The model under review builds one solid part; all positions refer to its coordinate system, in mm. Coordinates: 2 decimals unless noted, no trailing zeros. Loops run counter-clockwise (first coordinate to the right, second up) from the corner with the lowest first, then second, coordinate; pieces in that order, holes last. Notation, with made-up numbers: (50, 80) - (98, 80) arc R19 cw to (98, 88) - close; hole circle Ø1 at (32, 56). An arc over 180 degrees is marked (long way). One line per item, written item: value. Start each with the question number.
1. We need section A-A, the plane z = 111. Give the boundary of the cut face in (x, y).
2. We need section C-C, the plane y = -13.5. Give the boundary of the cut face in (x, z), then the cut area to 3 significant figures.
3. We need section B-B, the plane x = -7.25. Give the boundary of the cut face in (y, z), then the cut area to 3 significant figures.
4. Insertion check: P1, Ø4, axis at y = -15.5, z = 39, coming from the -X side. The pin has a flat end and moves straight along its axis. Give the tip position at first contact, or say it passes through.
5. To check wall thickness, follow line 1 (Y direction, x = 6.5, z = 116); line 2 (X direction, y = -5, z = 13.5); line 3 (X direction, y = -9, z = 130.5). State the ranges of each line that lie inside material, in increasing order.
Autodesk Inventor part; units mm, degrees
ref_plane "YZ Plane" through (0, 0, 0) normal (1, 0, 0) x (0, 1, 0)
ref_plane "XZ Plane" through (0, 0, 0) normal (0, 1, 0) x (-1, 0, 0)
ref_plane "XY Plane" through (0, 0, 0) normal (0, 0, 1) x (1, 0, 0)
sketch "Sketch1" plane through (0, 0, 0) normal (0, 0, 1) x (1, 0, 0)
  line L0 (-4.3602, -2.3462) -> (5.1648, -2.3462)
  line L1 (5.1648, -2.3462) -> (9.9273, -10.5951)
  line L2 (9.9273, -10.5951) -> (5.1648, -18.844)
  line L3 (5.1648, -18.844) -> (-4.3602, -18.844)
  line L4 (-4.3602, -18.844) -> (-9.1227, -10.5951)
  line L5 (-9.1227, -10.5951) -> (-4.3602, -2.3462)
  point P0 (0, 0)
  dimension "d0" = 9.525
  dimension "d1" = 9.525
  dimension "d2" = 9.525
  dimension "d3" = 9.525
  dimension "d4" = 9.525
  dimension "d6" = 9.525
  dimension "d7" = 120
  dimension "d8" = 120
  dimension "d9" = 120
  dimension "d10" = 120
  dimension "d11" = 120
extrude "Extrusion1" add sketch "Sketch1" along normal blind 157.48
properties part number "hex shaft"
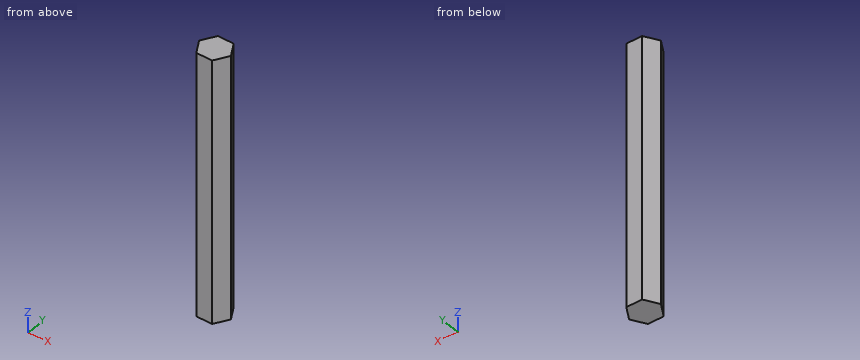
Findings below:
1. outline: (-9.12, -10.6) - (-4.36, -18.84) - (5.16, -18.84) - (9.93, -10.6) - (5.16, -2.35) - (-4.36, -2.35) - close
2. outline: (-7.45, 0) - (8.25, 0) - (8.25, 157.48) - (-7.45, 157.48) - close
2. area: 2,470 mm2
3. outline: (-13.84, 0) - (-7.35, 0) - (-7.35, 157.48) - (-13.84, 157.48) - close
3. area: 1,020 mm2
4. P1: x = -7.45
5. line 1: -16.53 to -4.66
5. line 2: -5.89 to 6.7
5. line 3: -8.2 to 9.01
